```python
from build123d import *

# Parameters (mm, degrees)
F0_R     = 9
F0_R_2   = 5.125
F1_DEPTH = 4.27
F0_R_3   = 3.625
F2_DEPTH = 6.9
F3_R     = 2


with BuildPart() as f1:
    # F0 (on Front) → F1 (new body)
    with BuildSketch(Plane.XZ):
        Circle(F0_R)
        Circle(F0_R_2, mode=Mode.SUBTRACT)
    extrude(amount=F1_DEPTH)

    # F0 (on Front) → F2 (join)
    with BuildSketch(Plane.XZ):
        Circle(F0_R_2)
        Circle(F0_R_3, mode=Mode.SUBTRACT)
    extrude(amount=F2_DEPTH)

    # F3
    f3_edges = [f1.edges().sort_by_distance(p)[0] for p in [
        (-9, -4.27, 0),
        (-9, 0, 0),
    ]]
    fillet(f3_edges, radius=F3_R)


solid = f1.part
```
Check sheet for the modelled part. Datum: model origin and axes. Units: mm. A direction names the side the tool comes from. Round coordinates to 2 decimals unless told otherwise and drop trailing zeros. Order: outer loops, then holes, each group sorted by start corner. A loop starts at its lowest first (then second) coordinate and runs counter-clockwise, first axis right, second up. Notation, with made-up numbers: (-28, -33.75) -> (-10, -33.75) arc R16 ccw to (-10, -29.75) -> close; hole circle Ø1 at (13.5, -7.5). An arc over 180 degrees is marked (long way). One line per item, written item: value. Start each with the question number.
Q1. Gauge pin test, flat ends, axial feed: pin 1 Ø1.5 at (x, y) = (1, -3) entering from +Z; pin 2 Ø3 at (x, z) = (2, -7) entering from -Y. Record the tip position at first contact, or that the pin passes through.
Q2. Set-up check for faces 4 (the face through (2.2, -6.9, -3.3)), 5 (the face through (4, -4.27, 4)): record each of +Z, -Z, +X, -X, +Y, -Y from which the full face is reachable in a straight line by a thin tool's end or side.
Q3. Thickness scan on line 1 (Z direction, x = 0, y = -5) (3 decimals); line 2 (Z direction, x = 0, y = -2.25) (3 decimals); line 3 (Y direction, x = 6.5, z = 0.75). Record the ranges inside material, lowest first.
Q4. Mould release check, pull along X, two halves, no side actions. Record for faces 1 (the face through (-1.111, -5.567, -5.003)), 2 (the face through (1.7, -3.4, -3.2)), 3 (the face through (3, 0, -3)): pulls with the +X half, pulls with the -X half, needs draft (parallel to the pull), parting line crosses it, or undercut.
Q5. Cross-section at D-D (y = -2.75). Record the boundary of the cut face in (x, z) (3 decimals), and give its area (3 significant figures).
Q6. Cross-section at B-B (z = 0). Record the boundary of the cut face in (x, y) (3 decimals), and give its area (3 significant figures).
Q7. Cross-section at C-C (y = -4.75). Record the boundary of the cut face in (x, z) (3 decimals).
Q8. Cross-section at A-A (x = 0). Record the boundary of the cut face in (y, z) (3 decimals), and give its area (3 significant figures).
Completed:
1. pin 1: stops at z = 8.98
1. pin 2: stops at y = -4.27
2. face 4: +Z, -Z, +X, -X, -Y
2. face 5: -Y
3. line 1: z = -5.125 to -3.625, 3.625 to 5.125
3. line 2: z = -9 to -3.625, 3.625 to 9
3. line 3: y = -4.27 to 0
4. face 1: parting line crosses it
4. face 2: undercut
4. face 3: needs draft
5. outline: circle Ø17.883 at (0, 0); hole circle Ø7.25 at (0, 0)
5. area: 210 mm²
6. outline: (-9, -2.27) arc R2 ccw to (-7, -4.27) -> (-5.125, -4.27) -> (-5.125, -6.9) -> (-3.625, -6.9) -> (-3.625, 0) -> (-7, 0) arc R2 ccw to (-9, -2) -> close; (3.625, -6.9) -> (5.125, -6.9) -> (5.125, -4.27) -> (7, -4.27) arc R2 ccw to (9, -2.27) -> (9, -2) arc R2 ccw to (7, 0) -> (3.625, 0) -> close
6. area: 50.4 mm²
7. outline: circle Ø10.25 at (0, 0); hole circle Ø7.25 at (0, 0)
8. outline: (-6.9, -5.125) -> (-4.27, -5.125) -> (-4.27, -7) arc R2 ccw to (-2.27, -9) -> (-2, -9) arc R2 ccw to (0, -7) -> (0, -3.625) -> (-6.9, -3.625) -> close; (-6.9, 3.625) -> (0, 3.625) -> (0, 7) arc R2 ccw to (-2, 9) -> (-2.27, 9) arc R2 ccw to (-4.27, 7) -> (-4.27, 5.125) -> (-6.9, 5.125) -> close
8. area: 50.4 mm²
